Build history of the part. All positions in model axes, mm. A direction names the side the tool comes from. Give positions to 0.01 mm unless a question says otherwise; leave off trailing zeros. Order: outer loops, then holes, each group sorted by start corner. A loop starts at its lowest first (then second) coordinate and runs counter-clockwise, first axis right, second up. Notation, with made-up numbers: (76.5, 14.5) - (126.5, 14.5) arc R20 cw to (126.5, 21.5) - close; hole circle Ø8 at (25, -29.75). An arc over 180 degrees is marked (long way). One line per item, written item: value.
```python
from build123d import *


with BuildPart() as part:
    # Sketch2 → Revolve1 (revolve)
    with BuildSketch(Plane(origin=(0, 0, 0), x_dir=(0, 0, -1), z_dir=(1, 0, 0)), mode=Mode.PRIVATE) as revolve1_sk:
        Polygon((-53.975, 63.896875), (53.975, 63.896875), (53.975, 57.15), (2.38125, 57.15), (2.38125, 50.8), (-2.38125, 50.8), (-2.38125, 57.15), (-53.975, 57.15), align=None)
    revolve(revolve1_sk.sketch.rotate(Axis((0, 0, 62.594581749), (0, 0, -1)), 90), axis=Axis((0, 0, 62.594581749), (0, 0, -1)))  # turned: the seam where the file's is


solid = part.part
```
(1) Pull direction Y, two halves, no side cores. Call faces 4 (the face through (29.48, 56.69, -0.76)), 5 (the face through (-48, 33, -53.975)), 6 (the face through (-57.095, -2.513, -27.817)): +Y half, -Y half, draft (parallel to the pull), parting line (faces both ways), or undercut.
Completed:
face 4: parting line
face 5: draft
face 6: undercut
(2) Pin check, flat tips, straight feed: P1, Ø3, axis at x = 48.5, y = -16.5, coming from the -Z side; P2, Ø1, axis at x = 15.5, z = -5.5, coming from the +Y side; P3, Ø6, axis at y = -32.5, z = 13, coming from the -X side. Stop position of each tip, or through.
Completed:
P1: z = -2.38
P2: y = 62.11
P3: x = -56.68
(3) Slice it at A-A, the plane x = 0. Give the cut face in (y, z) (3 decimals).
Completed:
outline: (-63.897, -53.975) - (-57.15, -53.975) - (-57.15, -2.381) - (-50.8, -2.381) - (-50.8, 2.381) - (-57.15, 2.381) - (-57.15, 53.975) - (-63.897, 53.975) - close; (50.8, -2.381) - (57.15, -2.381) - (57.15, -53.975) - (63.897, -53.975) - (63.897, 53.975) - (57.15, 53.975) - (57.15, 2.381) - (50.8, 2.381) - close
(4) Drill centre lines: line 1 (X direction, y = 0.5, z = 5.5); line 2 (Y direction, x = 0, z = 28.5); line 3 (Y direction, x = 0, z = 0). Where is each one in solid material? Low to high.
Completed:
line 1: -63.89 to -57.15, 57.15 to 63.89
line 2: -63.9 to -57.15, 57.15 to 63.9
line 3: -63.9 to -50.8, 50.8 to 63.9
(5) 3-axis set-ups, long thin cutter, end or side, ignore diameter. For faces 1 (the face through (48, 33, 53.975)), 2 (the face through (-38, 34, -2.381)), 3 (the face through (-57.095, -2.513, 28.539)): which of +Z, -Z, +X, -X, +Y, -Y reach the whole face in a straight line?
Completed:
face 1: +Z, +X, -X, +Y, -Y
face 2: -Z
face 3: +Z
(6) Slice it at C-C, the plane z = 34. Give the cut face in (x, y), and give its area (3 significant figures).
Completed:
outline: circle Ø127.79 at (0, 0); hole circle Ø114.3 at (0, 0)
area: 2,570 mm²
